Geometry: final body of the model. Coordinates: model frame, mm. A direction names the side the tool comes from. Give positions to 0.01 mm unless a question says otherwise; leave off trailing zeros. Order: outer loops, then holes, each group sorted by start corner. A loop starts at its lowest first (then second) coordinate and runs counter-clockwise, first axis right, second up. Notation, with made-up numbers: M 53.5,-6.75 L 107.5,-6.75 A24 ccw 107.5,27.25 Z; hole C 65,14 d10. An arc over 180 degrees is marked long. Write item = value, one per line. Start each with the question number.
from build123d import *

# Parameters (mm, degrees)
SKETCH_1_W           = 42
SKETCH_1_H           = 42
EXTRUDE_1_DEPTH      = 33
CUT_EXTRUDE_START    = 33
CUT_EXTRUDE_1_DEPTH  = 33
CUT_EXTRUDE_START_2  = 9.5
CUT_EXTRUDE_2_DEPTH  = 16
CUT_EXTRUDE_START_3  = 21
SKETCH_4_W           = 33
SKETCH_4_H           = 16
CUT_EXTRUDE_3_DEPTH  = 0.1
CUT_EXTRUDE_START_4  = -21
SKETCH_5_W           = 33
SKETCH_5_H           = 16
CUT_EXTRUDE_4_DEPTH  = 0.1
SKETCH_6_W           = 33
SKETCH_6_H           = 16
CUT_EXTRUDE_5_DEPTH  = 0.1
SKETCH_7_W           = 33
SKETCH_7_H           = 16
CUT_EXTRUDE_6_DEPTH  = 0.1
SKETCH_8_R           = 4.75
CUT_EXTRUDE_7_DEPTH  = 3
EXTRUDE_START        = 33
SKETCH_9_R           = 11
EXTRUDE_2_DEPTH      = 2
CUT_EXTRUDE_START_5  = 35
SKETCH_11_R          = 2.5
CUT_EXTRUDE_8_DEPTH  = 35
SKETCH_12_R          = 1.5
CUT_EXTRUDE_9_DEPTH  = 33
EXTRUDE_START_2      = 21
SKETCH_13_W          = 15.3
SKETCH_13_H          = 2.2
EXTRUDE_3_DEPTH      = 4
SKETCH_17_W          = 15.3
SKETCH_17_H          = 5.5
EXTRUDE_7_DEPTH      = 4
CUT_EXTRUDE_START_6  = 25
CUT_EXTRUDE_11_DEPTH = 4
EXTRUDE_START_3      = 7.65
EXTRUDE_8_DEPTH      = 15.3


with BuildPart() as part:
    # 草图1 → 凸台-拉伸1 (new body)
    with BuildSketch(Plane(origin=(0, 0, 0), x_dir=(1, 0, 0), z_dir=(0, 1, 0))):
        Rectangle(SKETCH_1_W, SKETCH_1_H)
    extrude(amount=EXTRUDE_1_DEPTH)

    # 草图2 → 切除-拉伸1 (cut)
    with BuildSketch(Plane(origin=(0, 0, 0), x_dir=(1, 0, 0), z_dir=(0, 1, 0)).offset(CUT_EXTRUDE_START)):
        Polygon((-21, 21), (-21, 16.5), (-16.5, 21), align=None)
        Polygon((-21, -21), (-21, -16.5), (-16.5, -21), align=None)
        Polygon((21, -21), (21, -16.5), (16.5, -21), align=None)
        Polygon((21, 21), (21, 16.5), (16.5, 21), align=None)
    extrude(amount=-CUT_EXTRUDE_1_DEPTH, mode=Mode.SUBTRACT)

    # 草图3 → 切除-拉伸2 (cut)
    with BuildSketch(Plane(origin=(0, 0, 0), x_dir=(1, 0, 0), z_dir=(0, 1, 0)).offset(CUT_EXTRUDE_START_2)):
        Polygon((-21, 13.5), (-21, 21), (-13.5, 21), align=None)
        Polygon((-21, -13.5), (-21, -21), (-13.5, -21), align=None)
        Polygon((21, -13.5), (21, -21), (13.5, -21), align=None)
        Polygon((21, 13.5), (21, 21), (13.5, 21), align=None)
    extrude(amount=CUT_EXTRUDE_2_DEPTH, mode=Mode.SUBTRACT)

    # 草图4 → 切除-拉伸3 (cut)
    with BuildSketch(Plane.XY.offset(CUT_EXTRUDE_START_3)):
        with Locations((0, 17.5)):
            Rectangle(SKETCH_4_W, SKETCH_4_H)
    extrude(amount=-CUT_EXTRUDE_3_DEPTH, mode=Mode.SUBTRACT)

    # 草图5 → 切除-拉伸4 (cut)
    with BuildSketch(Plane.XY.offset(CUT_EXTRUDE_START_4)):
        with Locations((0, 17.5)):
            Rectangle(SKETCH_5_W, SKETCH_5_H)
    extrude(amount=CUT_EXTRUDE_4_DEPTH, mode=Mode.SUBTRACT)

    # 草图6 → 切除-拉伸5 (cut)
    with BuildSketch(Plane(origin=(0, 0, 0), x_dir=(0, 0, -1), z_dir=(1, 0, 0)).offset(CUT_EXTRUDE_START_4)):
        with Locations((0, 17.5)):
            Rectangle(SKETCH_6_W, SKETCH_6_H)
    extrude(amount=CUT_EXTRUDE_5_DEPTH, mode=Mode.SUBTRACT)

    # 草图7 → 切除-拉伸6 (cut)
    with BuildSketch(Plane(origin=(0, 0, 0), x_dir=(0, 0, -1), z_dir=(1, 0, 0)).offset(CUT_EXTRUDE_START_3)):
        with Locations((0, 17.5)):
            Rectangle(SKETCH_7_W, SKETCH_7_H)
    extrude(amount=-CUT_EXTRUDE_6_DEPTH, mode=Mode.SUBTRACT)

    # 草图8 → 切除-拉伸7 (cut)
    with BuildSketch(Plane(origin=(0, 0, 0), x_dir=(1, 0, 0), z_dir=(0, 1, 0))):
        with Locations(Location((0, 0, 0), (0, 0, 90))):
            Circle(SKETCH_8_R)
    extrude(amount=CUT_EXTRUDE_7_DEPTH, mode=Mode.SUBTRACT)

    # 草图9 → 凸台-拉伸2 (add)
    with BuildSketch(Plane(origin=(0, 0, 0), x_dir=(1, 0, 0), z_dir=(0, 1, 0)).offset(EXTRUDE_START)):
        with Locations(Location((0, 0, 0), (0, 0, 90))):
            Circle(SKETCH_9_R)
    extrude(amount=EXTRUDE_2_DEPTH)

    # 草图11 → 切除-拉伸8 (cut)
    with BuildSketch(Plane(origin=(0, 0, 0), x_dir=(1, 0, 0), z_dir=(0, 1, 0)).offset(CUT_EXTRUDE_START_5)):
        with Locations(Location((0, 0, 0), (0, 0, 90))):
            Circle(SKETCH_11_R)
    extrude(amount=-CUT_EXTRUDE_8_DEPTH, mode=Mode.SUBTRACT)

    # 草图12 → 切除-拉伸9 (cut)
    with BuildSketch(Plane(origin=(0, 0, 0), x_dir=(1, 0, 0), z_dir=(0, 1, 0)).offset(CUT_EXTRUDE_START)):
        with Locations(Location((-15.5, 15.5, 0), (0, 0, 90))):
            Circle(SKETCH_12_R)
        with Locations(Location((-15.5, -15.5, 0), (0, 0, 90))):
            Circle(SKETCH_12_R)
        with Locations(Location((15.5, -15.5, 0), (0, 0, 90))):
            Circle(SKETCH_12_R)
        with Locations(Location((15.5, 15.5, 0), (0, 0, 90))):
            Circle(SKETCH_12_R)
    extrude(amount=-CUT_EXTRUDE_9_DEPTH, mode=Mode.SUBTRACT)

    # 草图13 → 凸台-拉伸3 (add)
    with BuildSketch(Plane.XY.offset(EXTRUDE_START_2)):
        with Locations((0, 1.1)):
            Rectangle(SKETCH_13_W, SKETCH_13_H)
    extrude(amount=EXTRUDE_3_DEPTH)

    # 草图17 → 凸台-拉伸7 (add)
    with BuildSketch(Plane.XY.offset(EXTRUDE_START_2)):
        with Locations((0, 6.75)):
            Rectangle(SKETCH_17_W, SKETCH_17_H)
    extrude(amount=EXTRUDE_7_DEPTH)

    # 草图18 → 切除-拉伸11 (cut)
    with BuildSketch(Plane.XY.offset(CUT_EXTRUDE_START_6)):
        Polygon((-6.65, 8.5), (-4, 8.5), (-4, 9.5), (4, 9.5), (4, 8.5), (6.65, 8.5), (6.65, 5), (-6.65, 5), align=None)
    extrude(amount=-CUT_EXTRUDE_11_DEPTH, mode=Mode.SUBTRACT)

    # 草图19 → 凸台-拉伸8 (add)
    with BuildSketch(Plane(origin=(0, 0, 0), x_dir=(0, 0, -1), z_dir=(1, 0, 0)).offset(EXTRUDE_START_3)):
        Polygon((-21, 9.5), (-20.9, 9.5), (-20.9, 9.6), align=None)
    extrude(amount=-EXTRUDE_8_DEPTH)


solid = part.part
1) Cut plane D-D (z = 0). Return loops of the section in (x, y), plus the area to 3 significant figures.
2) Cut plane A-A (z = -15.5). Return loops of the section in (x, y), plus the area to 3 significant figures.
3) Draft query along Y for faces 4 (the flat face through (0, 1, 25)), 5 (the flat face through (0, 7, 21)). Return one class per face: pulls with the +Y half, pulls with the -Y half, needs draft (parallel to the pull), parting line crosses it, or undercut.
4) Cut plane C-C (x = 15.5). Return loops of the section in (y, z), plus the area to 3 significant figures.
5) Cut plane B-B (y = 27.5). Return loops of the section in (x, z), plus the area to 3 significant figures.
6) Pin query (flat end, axial travel): pin 1 Ø1.8 at (x, z) = (15.5, 15.5) entering from +Y; pin 2 Ø0.7 at (y, z) = (1.5, 24) entering from -X; pin 3 Ø3.5 at (x, y) = (2, 8) entering from +Z; pin 4 Ø2 at (y, z) = (18.5, 18.5) entering from +X. Return the tip coordinate at first contact, or that it passes through.
7) Ray query, L1, parallel to X at y = 7.5, z = -15.5; L2, parallel to Z at x = 15.5, y = 18.5. Return the intervals inside material, ascending.
8) Access query for faces 1 (the flat face through (20.9, 18, 0)), 2 (the flat face through (-17.2, 17.4, 17.3)), 3 (the flat face through (-5, 8.5, 23)). Directions: +Z, -Z, +X, -X, +Y, -Y. A direction counts if a zero-diameter tool reaches every point of the face in a straight line with its end or side. Return the directions, or none.
Reply:
q1.outline = M -21,0 L -4.75,0 L -4.75,3 L -2.5,3 L -2.5,35 L -11,35 L -11,33 L -21,33 L -21,25.5 L -20.9,25.5 L -20.9,9.5 L -21,9.5 Z; M 2.5,3 L 4.75,3 L 4.75,0 L 21,0 L 21,9.5 L 20.9,9.5 L 20.9,25.5 L 21,25.5 L 21,33 L 11,33 L 11,35 L 2.5,35 Z
q1.area = 1,240 mm²
q2.outline = M -21,0 L -17,0 L -17,33 L -21,33 L -21,25.5 L -19,25.5 L -19,9.5 L -21,9.5 Z; M -14,0 L 14,0 L 14,33 L -14,33 Z; M 17,0 L 21,0 L 21,9.5 L 19,9.5 L 19,25.5 L 21,25.5 L 21,33 L 17,33 Z
q2.area = 1,120 mm²
q3.face_4 = needs draft
q3.face_5 = undercut
q4.outline = M 0,-21 L 9.5,-21 L 9.5,-19 L 25.5,-19 L 25.5,-21 L 33,-21 L 33,-17 L 0,-17 Z; M 0,-14 L 33,-14 L 33,14 L 0,14 Z; M 0,17 L 33,17 L 33,21 L 25.5,21 L 25.5,19 L 9.5,19 L 9.5,21 L 0,21 Z
q4.area = 1,120 mm²
q5.outline = M -21,-16.5 L -16.5,-21 L 16.5,-21 L 21,-16.5 L 21,16.5 L 16.5,21 L -16.5,21 L -21,16.5 Z; hole C -15.5,-15.5 d3; hole C -15.5,15.5 d3; hole C 0,0 d5; hole C 15.5,-15.5 d3; hole C 15.5,15.5 d3
q5.area = 1,680 mm²
q6.pin_1 = through
q6.pin_2 = -7.65
q6.pin_3 = 21
q6.pin_4 = 17
q7.L1 = -21 to -17, -14 to 14, 17 to 21
q7.L2 = -19 to -17, -14 to 14, 17 to 19
q8.face_1 = +Z, -Z, +X
q8.face_2 = +Z, -X
q8.face_3 = +Z
